Input: dimensioned drawing with shaded views. Units: mm. Origin: part minimum x, y, z. A direction names the side the tool comes from. Coordinates: 2 decimals unless noted, no trailing zeros. Loops run counter-clockwise (first coordinate to the right, second up) from the corner with the lowest first, then second, coordinate; pieces in that order, holes last.
(1) Set-up query: the marked faces 1, 2 and 3. Return all of +Z, -Z, +X, -X, +Y, -Y with unobstructed straight access to the full face (end or side cutting, diameter ignored); none if empty.
(2) Section B-B, the plane x = 12.5. Return loops of the section in (y, z).
(3) Line query: L1, parallel to Y at x = 17.5, z = 162.5; L2, parallel to Z at x = 3.5, y = 6; L3, parallel to Z at x = 21, y = 15.75. Output: solid intervals per line, ascending.
(4) Contact query for flat-ended pins moving along their axis: P1, Ø9, axis at y = 12.5, z = 162.5, coming from the -X side; P2, Ø12, axis at x = 17.5, z = 35.5, coming from the -Y side. Output: stop coordinate, or through.
(5) Section D-D, the plane z = 63. Return loops of the section in (x, y).
(6) Section A-A, the plane y = 12.5. Return loops of the section in (x, z), then the cut area to 4 significant figures.
(7) Section C-C, the plane z = 162.5. Return loops of the section in (x, y).
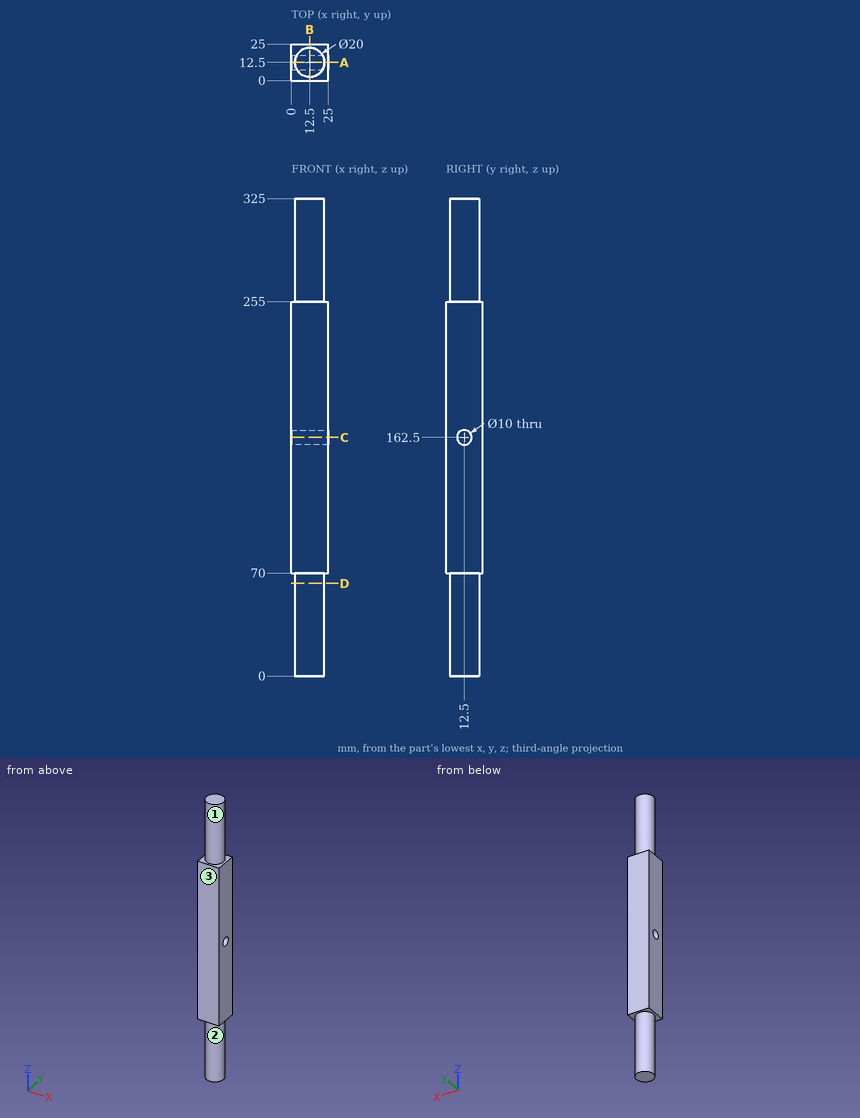
Report:
1. face 1: +Z
1. face 2: -Z
1. face 3: +Z, -Z, +X, -X, -Y
2. outline: (0, 70) - (2.5, 70) - (2.5, 0) - (22.5, 0) - (22.5, 70) - (25, 70) - (25, 255) - (22.5, 255) - (22.5, 325) - (2.5, 325) - (2.5, 255) - (0, 255) - close; hole circle Ø10 at (12.5, 162.5)
3. L1: y = 0 to 7.5, 17.5 to 25
3. L2: z = 70 to 255
3. L3: z = 0 to 158.7, 166.3 to 325
4. P1: passes through
4. P2: stops at y = 2.5
5. outline: circle Ø20 at (12.5, 12.5)
6. outline: (0, 70) - (2.5, 70) - (2.5, 0) - (22.5, 0) - (22.5, 70) - (25, 70) - (25, 157.5) - (0, 157.5) - close; (0, 167.5) - (25, 167.5) - (25, 255) - (22.5, 255) - (22.5, 325) - (2.5, 325) - (2.5, 255) - (0, 255) - close
6. area: 7,175 mm2
7. outline: (0, 0) - (25, 0) - (25, 7.5) - (0, 7.5) - close; (0, 17.5) - (25, 17.5) - (25, 25) - (0, 25) - close
